Study the drawing (mm; zero at the part's minimum x, y, z) and answer. A direction names the side the tool comes from. Coordinates: 2 decimals unless noted, no trailing zeros. Order: outer loops, then holes, each group sorted by start corner. A loop starts at its lowest first (then second) coordinate and runs counter-clockwise, first axis right, second up. Notation, with made-up numbers: M 63.25,-20.5 L 67.25,-20.5 A31 cw 67.25,11.5 Z; hole C 87,78.25 d2. An arc over 180 degrees is marked long. Use a Markdown table: item, result. Add a question column.
1) Find section D-D on x = 2108.2. Write down the section's boundary in (y, z), plus the area to 3 significant figures.
2) The mould has two halves that part along X. Classify the marked faces 1, 2 and 3: released by +X, released by -X, zero draft, split by the parting line, or undercut.
3) For the marked faces 4, 5, 6, 7 and 8, determine the directions among +Z, -Z, +X, -X, +Y, -Y from which every point of the face is accessible in a straight line to the end or side of a thin tool.
4) Find section B-B on y = 787.4. Write down the section's boundary in (x, z), plus the area to 3 significant figures.
5) Each of these flat-tipped pins is pushed along its axis until it touches: pin 1 Ø8 at (y, z) = (565, 420.5) entering from -X; pin 2 Ø5 at (y, z) = (873.5, 452.5) entering from +X; pin 3 Ø1.5 at (x, y) = (1927, 598) entering from +Z. Where does it stop, or does it pass through?
6) Find the intervals of material crossed by probe 1 along Y at (x, z) = (2108.2, 127); probe 2 along X at (y, z) = (228, 135); probe 3 along X at (y, z) = (663.5, 365.5), in increasing order. Write a range as [from, to].
7) Find section A-A on z = 125. Write down the section's boundary in (x, y).
8) Find section C-C on z = 348. Write down the section's boundary in (x, y).
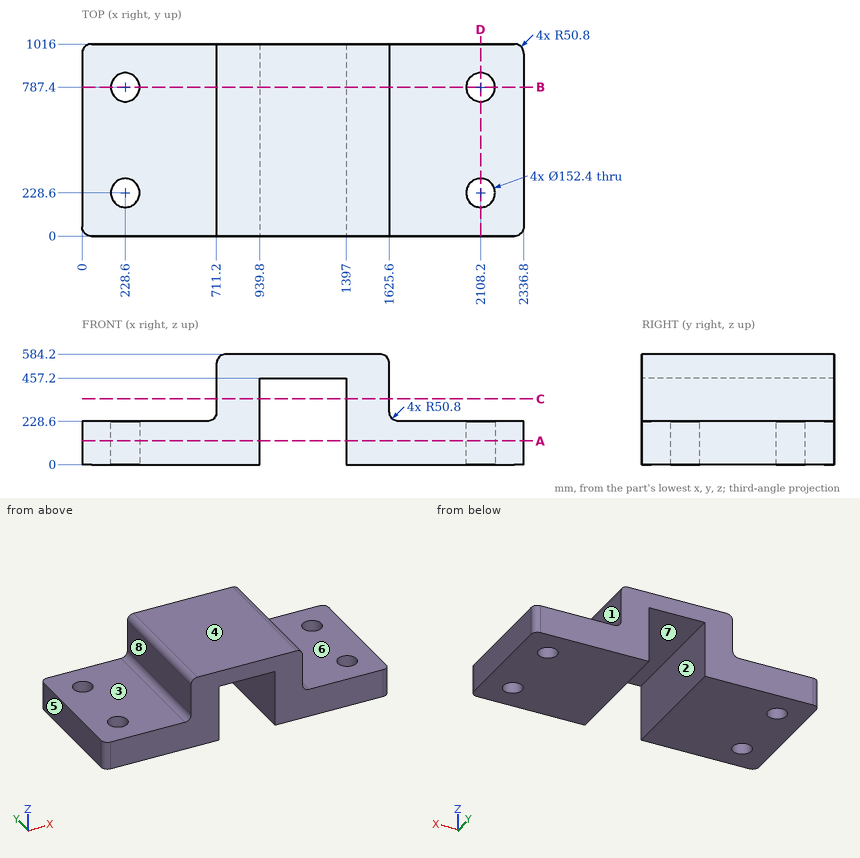
Check result:
| question | item | result |
|---|---|---|
| 1 | outline | M 0,0 L 152.4,0 L 152.4,228.6 L 0,228.6 Z; M 304.8,0 L 711.2,0 L 711.2,228.6 L 304.8,228.6 Z; M 863.6,0 L 1016,0 L 1016,228.6 L 863.6,228.6 Z |
| 1 | area | 163,000 mm2 |
| 2 | face 1 | released by +X |
| 2 | face 2 | undercut |
| 2 | face 3 | zero draft |
| 3 | face 4 | +Z, +X, -X, +Y, -Y |
| 3 | face 5 | +Z, -Z, -X, +Y, -Y |
| 3 | face 6 | +Z, +X, +Y, -Y |
| 3 | face 7 | -Z, +Y, -Y |
| 3 | face 8 | +Z, -X, +Y, -Y |
| 4 | outline | M 0,0 L 152.4,0 L 152.4,228.6 L 0,228.6 Z; M 304.8,0 L 939.8,0 L 939.8,457.2 L 1397,457.2 L 1397,0 L 2032,0 L 2032,228.6 L 1676.4,228.6 A50.8 cw 1625.6,279.4 L 1625.6,533.4 A50.8 ccw 1574.8,584.2 L 762,584.2 A50.8 ccw 711.2,533.4 L 711.2,279.4 A50.8 cw 660.4,228.6 L 304.8,228.6 Z; M 2184.4,0 L 2336.8,0 L 2336.8,228.6 L 2184.4,228.6 Z |
| 4 | area | 581,000 mm2 |
| 5 | pin 1 | stops at x = 711.2 |
| 5 | pin 2 | stops at x = 1625.6 |
| 5 | pin 3 | stops at z = 228.6 |
| 6 | probe 1 | y = [0, 152.4], [304.8, 711.2], [863.6, 1016] |
| 6 | probe 2 | x = [0, 152.4], [304.8, 939.8], [1397, 2032], [2184.4, 2336.8] |
| 6 | probe 3 | x = [711.2, 939.8], [1397, 1625.6] |
| 7 | outline | M 0,50.8 A50.8 ccw 50.8,0 L 939.8,0 L 939.8,1016 L 50.8,1016 A50.8 ccw 0,965.2 Z; M 1397,0 L 2286,0 A50.8 ccw 2336.8,50.8 L 2336.8,965.2 A50.8 ccw 2286,1016 L 1397,1016 Z; hole C 228.6,228.6 d152.4; hole C 228.6,787.4 d152.4; hole C 2108.2,228.6 d152.4; hole C 2108.2,787.4 d152.4 |
| 8 | outline | M 711.2,0 L 939.8,0 L 939.8,1016 L 711.2,1016 Z; M 1397,0 L 1625.6,0 L 1625.6,1016 L 1397,1016 Z |
